from build123d import *

# Parameters (mm, degrees)
F0_R     = 1.5
F1_DEPTH = 3
F2_R     = 2.5
F3_DEPTH = 5
F4_R     = 1.15
F5_DEPTH = 10


with BuildPart() as f1:
    # F0 (on Front) → F1 (new body)
    with BuildSketch(Plane.XZ):
        with BuildLine():
            Line((-15.850437, 19.086891), (9.944777, 6.560055))
            ThreePointArc((9.944777, 6.560055), (13.448446, 6.553682), (15.202122, 9.586891))
            Line((15.202122, 9.586891), (15.202122, 24.086891))
            Line((15.202122, 24.086891), (-10.850437, 24.086891))
            Line((-10.850437, 24.086891), (-15.850437, 24.086891))
            Line((-15.850437, 24.086891), (-15.850437, 19.086891))
        make_face()
        with BuildLine():
            ThreePointArc((13.00116, 8.836891), (10.952122, 8.287853), (10.403084, 10.336891))
            ThreePointArc((10.403084, 10.336891), (12.090351, 11.035779), (13.202122, 9.586891))
            ThreePointArc((13.202122, 9.586891), (13.151011, 9.198662), (13.00116, 8.836891))
        make_face(mode=Mode.SUBTRACT)
        with Locations((-7.350437, 20.586891)):
            Circle(F0_R, mode=Mode.SUBTRACT)
    extrude(amount=F1_DEPTH)

    # F2 (on face) → F3 (join)
    with BuildSketch(Plane.XY.offset(24.086891)):
        with Locations((11.702122, 0)):
            Circle(F2_R)
        with Locations((-13.297878, 0)):
            Circle(F2_R)
    extrude(amount=-F3_DEPTH)

    # F4 (on face) → F5 (cut)
    with BuildSketch(Plane.XY.offset(24.086891)):
        with Locations((11.702122, 0)):
            Circle(F4_R)
        with Locations((-13.297878, 0)):
            Circle(F4_R)
    extrude(amount=-F5_DEPTH, mode=Mode.SUBTRACT)


with BuildPart() as f6_1:
    # F6: instance of F1
    add(f1.part.mirror(Plane.XZ))


solid = f6_1.part
Can you work these out from the model? Positions are in its coordinate system, mm. A direction names the side the tool comes from. Round coordinates to 2 decimals unless told otherwise and drop trailing zeros. Order: outer loops, then holes, each group sorted by start corner. A loop starts at its lowest first (then second) coordinate and runs counter-clockwise, first axis right, second up. Notation, with made-up numbers: (5.5, 1) -> (50.5, 1) arc R19 ccw to (50.5, 23) -> close; hole circle Ø5 at (41, 32). An arc over 180 degrees is marked (long way). Write each question's results on one line, items separated by ' | '. Start each with the question number.
Item 1: If we section it at D-D, the plane y = -1.8: Write out the boundary of the cut face in (x, z).
Item 2: Please list where these lines run through material, in increasing order: L1, parallel to X at y = 0.45, z = 20.5; L2, parallel to X at y = 0.95, z = 21.5; L3, parallel to X at y = 0.8, z = 19.
Item 3: If we section it at A-A, the plane y = 0.8: Write out the boundary of the cut face in (x, z).
Item 4: Will these pins go through, and if not, where does the flat tip stop? pin 1 (1.5 mm diameter, centred on x = 9.5, z = 11.5, fed in from -Y); pin 2 (1 mm diameter, centred on y = 0, z = 8.5, fed in from -X); pin 3 (2 mm diameter, centred on x = -13.3, y = 0, fed in from +Z); pin 4 (0.7 mm diameter, centred on x = -15.5, z = 21, fed in from -Y).
Item 5: If we section it at B-B, the plane z = 21.5: Write out the boundary of the cut face in (x, y).
Item 6: Thinking about a two-plate mould opening in X: for faces 6 (the flat face through (4, 0, 17)), 7 (the flat face through (-13.3, -1.3, 19.087)), 8 (the flat face through (15.202, 1, 17)), 9 (the flat face through (-3.13, 1.48, 12.91)), which applies, +X half, -X half, draft (parallel to the pull), parting line (faces both ways), or undercut?
Item 7: If we section it at C-C, the plane x = 12.5: Write out the boundary of the cut face in (y, z), then the cut area to 3 significant figures.
Item 8: Which directions (+Z, -Z, +X, -X, +Y, -Y) give clear straight access to the entire face, cutting with the end or side of a thin tool? Please do faces 1 (the cylindrical face through (11.45, 1.12, 20.27)), 2 (the flat face through (-1, 1, 24.087)), 3 (the flat face through (11.7, 0.4, 14.087)), 4 (the flat face through (11.7, -1.3, 19.087)), 5 (the cylindrical face through (13.404, 1.479, 6.528)).
Results:
1) outline: (-15.03, 19.09) -> (-11.56, 19.09) -> (-11.56, 24.09) -> (-15.03, 24.09) -> close; (9.97, 19.09) -> (13.44, 19.09) -> (13.44, 24.09) -> (9.97, 24.09) -> close
2) L1: x = -15.85 to -14.36, -12.24 to -8.85, -5.85 to 10.64, 12.76 to 15.2 | L2: x = -15.85 to -13.95, -12.65 to -8.54, -6.16 to 11.05, 12.35 to 15.2 | L3: x = -15.67 to -14.12, -12.47 to 10.88, 12.53 to 15.2
3) outline: (-15.85, 19.09) -> (-14.12, 18.25) -> (-14.12, 24.09) -> (-15.85, 24.09) -> close; (-12.47, 17.45) -> (9.94, 6.56) arc R3.5 ccw to (15.2, 9.59) -> (15.2, 24.09) -> (12.53, 24.09) -> (12.53, 14.09) -> (10.88, 14.09) -> (10.88, 24.09) -> (-12.47, 24.09) -> close; hole circle Ø3 at (-7.35, 20.59); hole (13, 8.84) arc R1.5 ccw to (13.2, 9.59) arc R1.5 ccw (long way) to start
4) pin 1: stops at y = 0 | pin 2: stops at x = 4.92 | pin 3: passes through | pin 4: stops at y = -1.68
5) outline: (-15.85, 0) -> (-15.8, 0) arc R2.5 ccw to (-10.8, 0) -> (-8.54, 0) -> (-8.54, 3) -> (-15.85, 3) -> close; (-6.16, 0) -> (9.2, 0) arc R2.5 ccw to (14.2, 0) -> (15.2, 0) -> (15.2, 3) -> (-6.16, 3) -> close; hole circle Ø2.3 at (-13.3, 0); hole circle Ø2.3 at (11.7, 0)
6) face 6: undercut | face 7: draft | face 8: +X half | face 9: -X half
7) outline: (-2.37, 19.09) -> (-0.83, 19.09) -> (-0.83, 24.09) -> (-2.37, 24.09) -> close; (0, 6.18) -> (3, 6.18) -> (3, 8.32) -> (0, 8.32) -> close; (0, 10.86) -> (3, 10.86) -> (3, 24.09) -> (0.83, 24.09) -> (0.83, 14.09) -> (0, 14.09) -> close | area: 45.5 mm2
8) face 1: +Z | face 2: +Z, +X, -X, +Y, -Y | face 3: +Z, -Y | face 4: -Z, +X, -X, -Y | face 5: -Z, +Y, -Y
